from build123d import *

# Parameters (mm, degrees)
SKETCH1_R           = 1.75
BOSS_EXTRUDE1_DEPTH = 4


with BuildPart() as part:
    # Sketch1 → Boss-Extrude1 (new body)
    with BuildSketch(Plane(origin=(0, 4, 0), x_dir=(1, 0, 0), z_dir=(0, 1, 0))):
        with BuildLine():
            Line((1.305695063, -4), (30.3065745, -4))
            ThreePointArc((30.3065745, -4), (34.3065745, 0), (30.3065745, 4))
            Line((30.3065745, 4), (2.081641936, 4))
            ThreePointArc((2.081641936, 4), (2.861028333, 4.588201733), (3.521749436, 5.30713988))
            ThreePointArc((3.521749436, 5.30713988), (3.405395609, 5.596745198), (3.282888305, 5.883801663))
            ThreePointArc((3.282888305, 5.883801663), (1.93527598, 5.894040025), (0.627094961, 5.57027124))
            ThreePointArc((0.627094961, 5.57027124), (0.366286148, 6.046375), (0.084372603, 6.510293938))
            ThreePointArc((0.084372603, 6.510293938), (1.018855105, 7.48132754), (1.683794586, 8.65351323))
            ThreePointArc((1.683794586, 8.65351323), (1.496450048, 8.903135899), (1.303821399, 9.148703928))
            ThreePointArc((1.303821399, 9.148703928), (-0.000522033, 8.809805691), (-1.180330337, 8.158486898))
            ThreePointArc((-1.180330337, 8.158486898), (-1.555477026, 8.550865528), (-1.947855656, 8.926012217))
            ThreePointArc((-1.947855656, 8.926012217), (-1.296536862, 10.105820521), (-0.957638625, 11.410163953))
            ThreePointArc((-0.957638625, 11.410163953), (-1.203206655, 11.602792602), (-1.452829324, 11.79013714))
            ThreePointArc((-1.452829324, 11.79013714), (-2.625015014, 11.125197659), (-3.596048616, 10.190715157))
            ThreePointArc((-3.596048616, 10.190715157), (-4.059967554, 10.472628702), (-4.536071314, 10.733437515))
            ThreePointArc((-4.536071314, 10.733437515), (-4.212302529, 12.041618533), (-4.222540891, 13.389230859))
            ThreePointArc((-4.222540891, 13.389230859), (-4.509597355, 13.511738163), (-4.799202674, 13.62809199))
            ThreePointArc((-4.799202674, 13.62809199), (-5.759348103, 12.682425791), (-6.455432668, 11.528463019))
            ThreePointArc((-6.455432668, 11.528463019), (-6.976508546, 11.680699536), (-7.503891752, 11.809396783))
            ThreePointArc((-7.503891752, 11.809396783), (-7.529737283, 13.156800143), (-7.888414517, 14.455843809))
            ThreePointArc((-7.888414517, 14.455843809), (-8.197396993, 14.499881098), (-8.507248835, 14.537314892))
            ThreePointArc((-8.507248835, 14.537314892), (-9.18992168, 13.375367565), (-9.563620196, 12.080565177))
            ThreePointArc((-9.563620196, 12.080565177), (-10.106342554, 12.09275), (-10.649064912, 12.080565177))
            ThreePointArc((-10.649064912, 12.080565177), (-11.022763428, 13.375367565), (-11.705436272, 14.537314892))
            ThreePointArc((-11.705436272, 14.537314892), (-12.015288115, 14.499881098), (-12.324270591, 14.455843809))
            ThreePointArc((-12.324270591, 14.455843809), (-12.682947825, 13.156800143), (-12.708793355, 11.809396783))
            ThreePointArc((-12.708793355, 11.809396783), (-13.236176561, 11.680699536), (-13.757252439, 11.528463019))
            ThreePointArc((-13.757252439, 11.528463019), (-14.453337005, 12.682425791), (-15.413482434, 13.62809199))
            ThreePointArc((-15.413482434, 13.62809199), (-15.703087752, 13.511738163), (-15.990144217, 13.389230859))
            ThreePointArc((-15.990144217, 13.389230859), (-16.000382579, 12.041618533), (-15.676613793, 10.733437515))
            ThreePointArc((-15.676613793, 10.733437515), (-16.152717554, 10.472628702), (-16.616636492, 10.190715157))
            ThreePointArc((-16.616636492, 10.190715157), (-17.587670094, 11.125197659), (-18.759855783, 11.79013714))
            ThreePointArc((-18.759855783, 11.79013714), (-19.009478453, 11.602792602), (-19.255046482, 11.410163953))
            ThreePointArc((-19.255046482, 11.410163953), (-18.916148245, 10.105820521), (-18.264829452, 8.926012217))
            ThreePointArc((-18.264829452, 8.926012217), (-18.657208082, 8.550865528), (-19.032354771, 8.158486898))
            ThreePointArc((-19.032354771, 8.158486898), (-20.212163074, 8.809805691), (-21.516506507, 9.148703928))
            ThreePointArc((-21.516506507, 9.148703928), (-21.709135156, 8.903135899), (-21.896479694, 8.65351323))
            ThreePointArc((-21.896479694, 8.65351323), (-21.231540213, 7.48132754), (-20.297057711, 6.510293938))
            ThreePointArc((-20.297057711, 6.510293938), (-20.578971255, 6.046375), (-20.839780068, 5.57027124))
            ThreePointArc((-20.839780068, 5.57027124), (-22.147961087, 5.894040025), (-23.495573413, 5.883801663))
            ThreePointArc((-23.495573413, 5.883801663), (-23.618080717, 5.596745198), (-23.734434544, 5.30713988))
            ThreePointArc((-23.734434544, 5.30713988), (-22.788768345, 4.346994451), (-21.634805572, 3.650909885))
            ThreePointArc((-21.634805572, 3.650909885), (-21.78704209, 3.129834008), (-21.915739337, 2.602450802))
            ThreePointArc((-21.915739337, 2.602450802), (-23.263142697, 2.576605271), (-24.562186363, 2.217928037))
            ThreePointArc((-24.562186363, 2.217928037), (-24.606223651, 1.908945561), (-24.643657446, 1.599093719))
            ThreePointArc((-24.643657446, 1.599093719), (-23.481710119, 0.916420874), (-22.186907731, 0.542722358))
            ThreePointArc((-22.186907731, 0.542722358), (-12.402167869, -11.872817218), (1.305695063, -4))
        make_face()
        with Locations(Location((30.3065745, 0, 0), (0, 0, 90))):
            Circle(SKETCH1_R, mode=Mode.SUBTRACT)
        with Locations(Location((-10.106342554, 0, 0), (0, 0, 90))):
            Circle(SKETCH1_R, mode=Mode.SUBTRACT)
    extrude(amount=-BOSS_EXTRUDE1_DEPTH)


solid = part.part
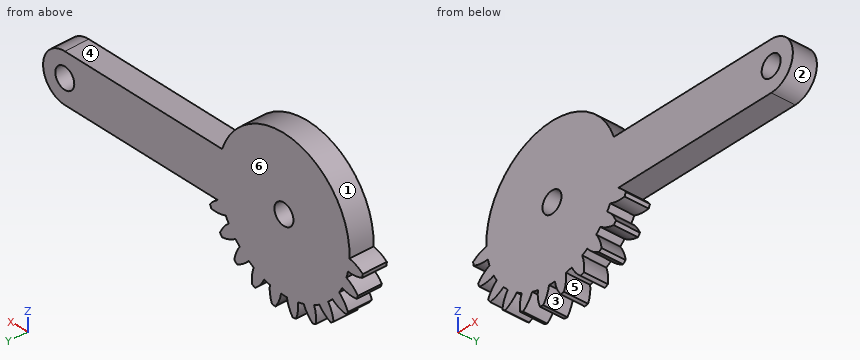
Verification items for the finished model (mm, model axes). Face numbers are marked on the shaded views. A direction names the side the tool comes from. Give positions to 0.01 mm unless a question says otherwise; leave off trailing zeros. Loops run counter-clockwise (first coordinate to the right, second up) from the corner with the lowest first, then second, coordinate; pieces in that order, holes last. Notation, with made-up numbers: (13, 34.25) - (35, 34.25) arc R22 ccw to (35, 69.25) - close; hole circle Ø3 at (8, 84.25). An arc over 180 degrees is marked (long way). Write each question's results on one line, items separated by ' | '.
1) Sectioned sample at B-B on x = 23. Record the boundary of the cut face in (y, z), plus the area to 3 significant figures.
Solution:
outline: (0, -4) - (4, -4) - (4, 4) - (0, 4) - close | area: 32.0 mm2
2) Depth check by flat-ended pin: P1, Ø1, axis at x = 0.5, y = 2.5, coming from the +Z side; P2, Ø4, axis at x = -10.11, z = 0, coming from the -Y side; P3, Ø2, axis at x = 14.5, y = 2, coming from the +Z side; P4, Ø1.2, axis at x = 20.5, y = 2, coming from the -Z side. Enter the tip coordinate at first touch or a pass-through.
Solution:
P1: z = 6.64 | P2: y = 0 | P3: z = 4 | P4: z = -4
3) Sectioned sample at C-C on y = 1.25. Count the separate pieces of the cut face and the enclosed holes in it, plus the area to 3 significant figures.
Solution:
separate pieces: 1 | enclosed holes: 2 | area: 738 mm2
4) Mould release check, pull along X, two halves, no side actions. Record for the marked faces 1, 2 and 3: pulls with the +X half, pulls with the -X half, needs draft (parallel to the pull), parting line crosses it, or undercut.
Solution:
face 1: parting line crosses it | face 2: pulls with the +X half | face 3: undercut
5) Material ranges on L1, parallel to X at y = 3.05, z = 0; L2, parallel to X at y = 0.35, z = 1; L3, parallel to Z at x = 23, y = 0.4, recorded low to high. Write a range as from..to.
Solution:
L1: -22.2..-11.86, -8.36..28.56, 32.06..34.31 | L2: -22.16..-11.54, -8.67..28.87, 31.74..34.18 | L3: -4..4
6) Tool access check on the marked faces 4, 5 and 6. Record the directions out of +Z, -Z, +X, -X, +Y, -Y that give a thin tool (end or side, any length) a straight path to the whole face; none if there is none.
Solution:
face 4: +Z, +X, +Y, -Y | face 5: +Y, -Y | face 6: +Z, -Z, +X, -X, +Y
7) Sectioned sample at A-A on z = 0. Record the boundary of the cut face in (x, y).
Solution:
outline: (-22.2, 0) - (-11.86, 0) - (-11.86, 4) - (-22.2, 4) - close; (-8.36, 0) - (28.56, 0) - (28.56, 4) - (-8.36, 4) - close; (32.06, 0) - (34.31, 0) - (34.31, 4) - (32.06, 4) - close
8) Sectioned sample at D-D on z = 7.5. Record the boundary of the cut face in (x, y), plus the area to 3 significant figures.
Solution:
outline: (-19.59, 0) - (-0.62, 0) - (-0.62, 4) - (-19.59, 4) - close | area: 75.9 mm2
